For this review, use the dimensioned drawing (mm, ordinates from the lowest corner) and the shaded views. A direction names the side the tool comes from. Give positions to 0.01 mm unless a question says otherwise; leave off trailing zeros. Order: outer loops, then holes, each group sorted by start corner. A loop starts at its lowest first (then second) coordinate and runs counter-clockwise, first axis right, second up. Notation, with made-up numbers: (24.5, 13.25) - (60.5, 13.25) arc R17 ccw to (60.5, 42.25) - close; hole circle Ø11 at (54.5, 39.5). An arc over 180 degrees is marked (long way). One line per item, written item: value.
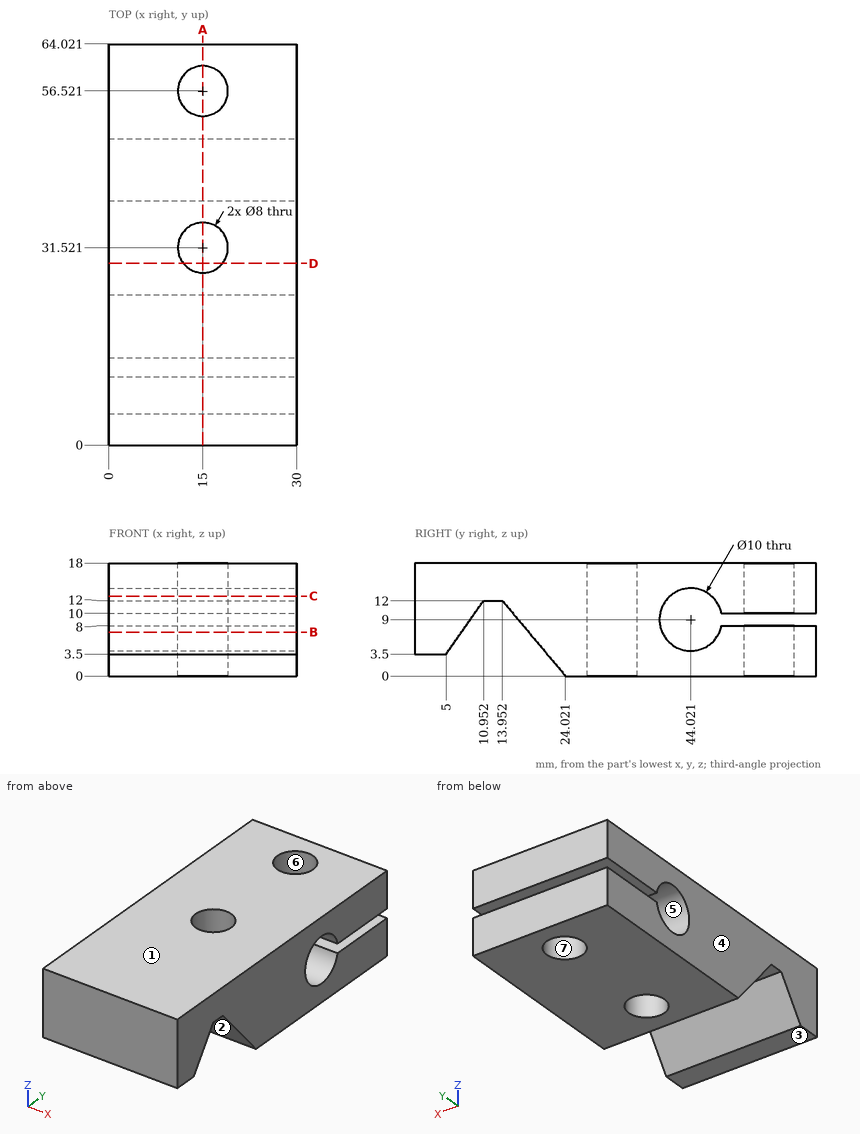
(1) Machinability: for the marked faces 1, 2 and 3, which of the approach directions +Z, -Z, +X, -X, +Y, -Y give a long, thin tool a straight path to every point of the face, cutting with its end or side? Answer none if there is none.
Answers below:
face 1: +Z, +X, -X, +Y, -Y
face 2: -Z, +X, -X
face 3: -Z, +X, -X, -Y
(2) For P1, Ø9, axis at y = 44.02, z = 9, coming from the +X side; P2, Ø1.5, axis at x = 20.5, y = 1.5, coming from the -Z side; P3, Ø3.5, axis at x = 18, y = 12.5, coming from the -Z side (1 decimal), all flat-tipped, find the tip position at first contact; note any pin that passes through.
Answers below:
P1: passes through
P2: stops at z = 3.5
P3: stops at z = 11.6
(3) Take a section at A-A (x = 15). Write out the cut boundary in (y, z), then the cut area to 3 significant figures.
Answers below:
outline: (0, 3.5) - (5, 3.5) - (10.95, 12) - (13.95, 12) - (24.02, 0) - (27.52, 0) - (27.52, 18) - (0, 18) - close; (35.52, 0) - (52.52, 0) - (52.52, 8) - (48.92, 8) arc R5 cw (long way) to (48.92, 10) - (52.52, 10) - (52.52, 18) - (35.52, 18) - close; (60.52, 0) - (64.02, 0) - (64.02, 8) - (60.52, 8) - close; (60.52, 10) - (64.02, 10) - (64.02, 18) - (60.52, 18) - close
area: 612 mm^2
(4) Draft analysis for pull direction X (two halves, no side actions). For the marked faces 4, 5, 6 and 7, state which applies: pulls with the +X half, pulls with the -X half, needs draft (parallel to the pull), parting line crosses it, or undercut.
Answers below:
face 4: pulls with the -X half
face 5: needs draft
face 6: undercut
face 7: undercut
(5) Take a section at B-B (z = 7). Write out the cut boundary in (x, y).
Answers below:
outline: (0, 0) - (30, 0) - (30, 7.45) - (0, 7.45) - close; (0, 18.15) - (30, 18.15) - (30, 39.44) - (0, 39.44) - close; (0, 48.6) - (30, 48.6) - (30, 64.02) - (0, 64.02) - close; hole circle Ø8 at (15, 31.52); hole circle Ø8 at (15, 56.52)
(6) Take a section at C-C (z = 12.75). Write out the cut boundary in (x, y), then the cut area to 3 significant figures.
Answers below:
outline: (0, 0) - (30, 0) - (30, 40.71) - (0, 40.71) - close; (0, 47.33) - (30, 47.33) - (30, 64.02) - (0, 64.02) - close; hole circle Ø8 at (15, 31.52); hole circle Ø8 at (15, 56.52)
area: 1,620 mm^2
(7) Take a section at D-D (y = 29). Write out the cut boundary in (x, z).
Answers below:
outline: (0, 0) - (11.89, 0) - (11.89, 18) - (0, 18) - close; (18.11, 0) - (30, 0) - (30, 18) - (18.11, 18) - close
(8) Wall thickness on line 1 (Z direction, x = 11.5, y = 51.5); line 2 (Y direction, x = 15, z = 14.25); line 3 (Y direction, x = 13, z = 10.25) (1 decimal): over which ranges is each line inside the solid? List them lowest first. Write a range as from..to.
Answers below:
line 1: z = 0..8, 10..18
line 2: y = 0..27.52, 35.52..52.52, 60.52..64.02
line 3: y = 0..9.7, 15.4..28.1, 35..39.2, 48.9..53.1, 60..64
